Answer from the drawing. Dimensions are ordinates in mm from the lowest x, y and z of the part. Round coordinates to 2 decimals unless told otherwise and drop trailing zeros. Order: outer loops, then holes, each group sorted by start corner. A loop starts at its lowest first (then second) coordinate and runs counter-clockwise, first axis right, second up.
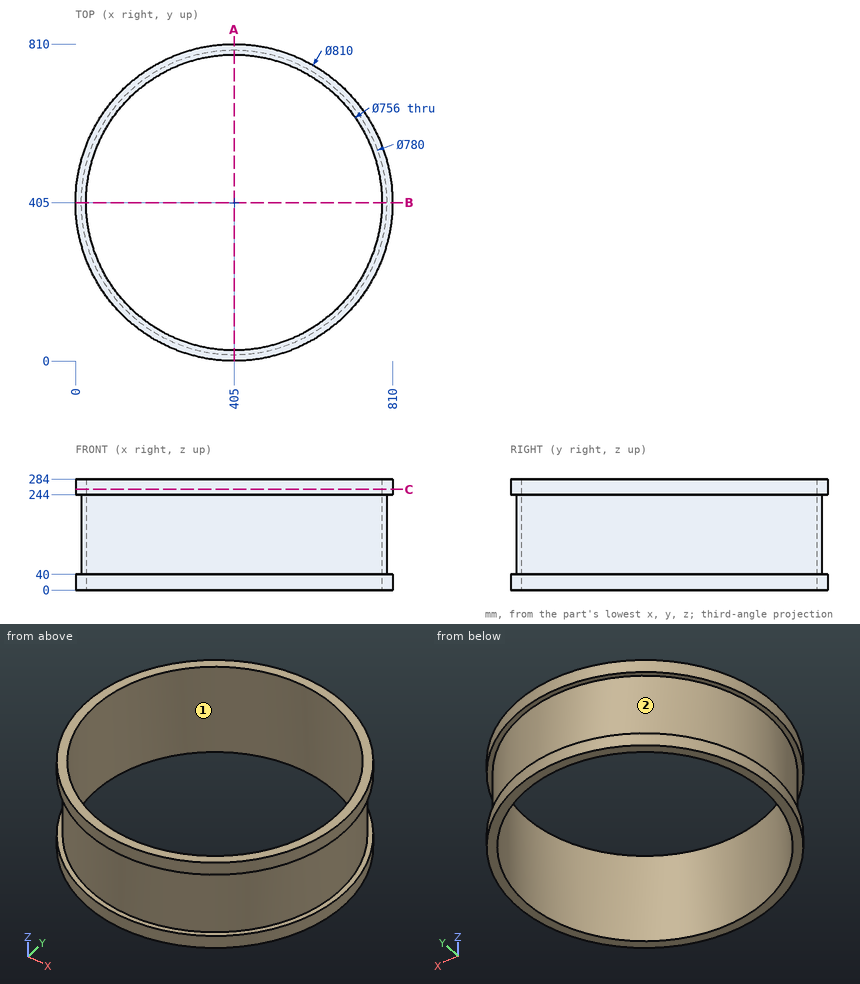
Q1. Flat-ended cylindrical pins translate along their axes: pin 1 (1.5 mm diameter, centred on x = 199, z = 162.5, fed in from +Y); pin 2 (6 mm diameter, centred on x = 479.5, z = 171, fed in from -Y); pin 3 (5 mm diameter, centred on x = 653, z = 79.5, fed in from -Y). Find the tip coordinate at first contact, or state that the pin passes through.
Outcome:
pin 1: stops at y = 736.62
pin 2: stops at y = 21.61
pin 3: stops at y = 101.97
Q2. A cutting plane is placed at C-C, the plane z = 257.5. Give the vertices of the cut face in (x, y), plus the area to 3 significant figures.
Outcome:
outline: circle Ø810 at (405, 405); hole circle Ø756 at (405, 405)
area: 66,400 mm2
Q3. Straight lines are drawn through the part: probe 1 along X at (y, z) = (405, 64.5); probe 2 along Z at (x, y) = (669, 106.5); probe 3 along X at (y, z) = (140.5, 21). For each, find the intervals that lie inside material, in ascending order.
Outcome:
probe 1: x = 15 to 27, 783 to 795
probe 2: z = 0 to 40, 244 to 284
probe 3: x = 98.3 to 134.96, 675.04 to 711.7
Q4. For a pull along Y with two mould halves and no side action, classify the marked faces 1 and 2 as released by +Y, released by -Y, zero draft, split by the parting line, or undercut.
Outcome:
face 1: undercut
face 2: split by the parting line
Q5. A cutting plane is placed at A-A, the plane x = 405. Give the vertices of the cut face in (y, z), plus the area to 3 significant figures.
Outcome:
outline: (0, 0) - (27, 0) - (27, 284) - (0, 284) - (0, 244) - (15, 244) - (15, 40) - (0, 40) - close; (783, 0) - (810, 0) - (810, 40) - (795, 40) - (795, 244) - (810, 244) - (810, 284) - (783, 284) - close
area: 9,220 mm2
